```python
from build123d import *

# Parameters (mm, degrees)
F0_W          = 1422.4
F0_H          = 711.2
F0_W_2        = 654.05
F0_H_2        = 635
F1_DEPTH      = 88.9
F2_W          = 88.9
F2_H          = 88.9
F3_DEPTH      = 762
F5_W          = 1422.4
F5_H          = 711.2
F5_W_2        = 654.05
F5_H_2        = 635
F6_DEPTH      = 88.9
F7_W          = 1422.4
F7_H          = 711.2
F8_DEPTH      = 18.796
F8_DEPTH_BACK = 0.254
F9_W          = 19.05
F9_H          = 533.4
F9_W_2        = 577.85
F9_H_2        = 19.05
F10_DEPTH     = 590.804
F12_W         = 152.4
F12_H         = 635
F13_DEPTH     = 88.9
F14_W         = 654.05
F14_H         = 635
F15_DEPTH     = 19.05


with BuildPart() as f1:
    # F0 (on Top) → F1 (new body)
    with BuildSketch(Plane.XY):
        with Locations((0, -355.6)):
            Rectangle(F0_W, F0_H)
        with Locations((-346.075, -355.6)):
            Rectangle(F0_W_2, F0_H_2, mode=Mode.SUBTRACT)
        with Locations((346.075, -355.6)):
            Rectangle(F0_W_2, F0_H_2, mode=Mode.SUBTRACT)
    extrude(amount=-F1_DEPTH)

    # F2 (on Top) → F3 (join)
    with BuildSketch(Plane.XY):
        with Locations((-666.75, -44.45)):
            Rectangle(F2_W, F2_H)
        with Locations((-666.75, -666.75)):
            Rectangle(F2_W, F2_H)
        with Locations((0, -44.45)):
            Rectangle(F2_W, F2_H)
        with Locations((0, -666.75)):
            Rectangle(F2_W, F2_H)
        with Locations((666.75, -44.45)):
            Rectangle(F2_W, F2_H)
        with Locations((666.75, -666.75)):
            Rectangle(F2_W, F2_H)
    extrude(amount=-F3_DEPTH)

    # F5 (on offset) → F6 (join)
    with BuildSketch(Plane.XY.offset(-609.6)):
        with Locations((0, -355.6)):
            Rectangle(F5_W, F5_H)
        with Locations((-346.075, -355.6)):
            Rectangle(F5_W_2, F5_H_2, mode=Mode.SUBTRACT)
        with Locations((346.075, -355.6)):
            Rectangle(F5_W_2, F5_H_2, mode=Mode.SUBTRACT)
    extrude(amount=-F6_DEPTH)

    # F7 (on offset) → F8 (join, two sides)
    with BuildSketch(Plane.XY.offset(-609.6)) as f8_sk:
        with Locations((0, -355.6)):
            Rectangle(F7_W, F7_H)
    extrude(amount=F8_DEPTH)
    extrude(f8_sk.sketch, amount=-F8_DEPTH_BACK)

    # F9 (on Top) → F10 (join, through all)
    with BuildSketch(Plane.XY):
        with Locations((663.575, -355.6)):
            Rectangle(F9_W, F9_H)
        with Locations((333.375, -47.625)):
            Rectangle(F9_W_2, F9_H_2)
        with Locations((-28.575, -355.6)):
            Rectangle(F9_W, F9_H)
        with Locations((-663.575, -355.6)):
            Rectangle(F9_W, F9_H)
    extrude(amount=-F10_DEPTH)

    # F12 (on offset) → F13 (join)
    with BuildSketch(Plane.XY.offset(-381)):
        Polygon((0, 0), (-711.2, 0), (-711.2, -38.1), (-542.925, -38.1), (-542.925, -673.1), (-711.2, -673.1), (-711.2, -711.2), (0, -711.2), (0, -673.1), (-123.825, -673.1), (-123.825, -38.1), (0, -38.1), align=None)
        with Locations((-428.625, -355.6)):
            Rectangle(F12_W, F12_H, mode=Mode.SUBTRACT)
        with Locations((-238.125, -355.6)):
            Rectangle(F12_W, F12_H, mode=Mode.SUBTRACT)
    extrude(amount=-F13_DEPTH)

    # F14 (on face) → F15 (join)
    with BuildSketch(Plane.XY.offset(-381)):
        with Locations((-346.075, -355.6)):
            Rectangle(F14_W, F14_H)
    extrude(amount=-F15_DEPTH)


solid = f1.part
```
Source: CAD feature listing. Evaluate the final solid. Frame: model axes, mm. A direction names the side the tool comes from. Coordinates: 2 decimals unless noted, no trailing zeros. Order: outer loops, then holes, each group sorted by start corner. A loop starts at its lowest first (then second) coordinate and runs counter-clockwise, first axis right, second up. Notation, with made-up numbers: M -8.75,-15 L 44.25,-15 A12 cw 44.25,7 Z; hole C -32.75,-24 d5. An arc over 180 degrees is marked long. Write each question's results on one line, items separated by ' | '. Start each with the question number.
1) Section query D-D (z = -659). Return the cut outline in (x, y).
2) Section query A-A (x = -568.5). Return the cut outline in (y, z), plus the area to 3 significant figures.
3) Line query: line 1 (X direction, y = -478.5, z = -590.5); line 2 (X direction, y = -154, z = -680.5); line 3 (Z direction, x = -591, y = -585.5). Output: solid intervals per line, ascending. Write a range as from..to.
4) Access query for faces 1 (the face through (692, -352, -88.9)), 2 (the face through (-19.05, -359, -336)), 3 (the face through (622.3, -55, -702)), 4 (the face through (329, -38.1, -336)). Directions: +Z, -Z, +X, -X, +Y, -Y. A direction counts if a zero-diameter tool reaches every point of the face in a straight line with its end or side. Return the directions, or none.
5) Section query C-C (z = -69). Return the cut outline in (x, y).
6) Section query B-B (x = 213). Return the cut outline in (y, z).
7) Contact query for flat-ended pins moving along their axis: pin 1 Ø5 at (y, z) = (-369.5, -137.5) entering from -X; pin 2 Ø3 at (x, y) = (-416.5, -218.5) entering from +Z; pin 3 Ø11.5 at (x, y) = (-368.5, -688.5) entering from -Z. Output: stop coordinate, or through.
8) Draft query along Y for faces 5 (the face through (-638, -88.9, -188)), 6 (the face through (-667, -44, -762)), 7 (the face through (-168, 0, -460)), 8 (the face through (622.3, -657, -702)). Return one class per face: released by +Y, released by -Y, zero draft, split by the parting line, or undercut.
Answers:
1) outline: M -711.2,-711.2 L 711.2,-711.2 L 711.2,0 L -711.2,0 Z; hole M -673.1,-622.3 L -622.3,-622.3 L -622.3,-673.1 L -44.45,-673.1 L -44.45,-622.3 L -19.05,-622.3 L -19.05,-88.9 L -44.45,-88.9 L -44.45,-38.1 L -622.3,-38.1 L -622.3,-88.9 L -673.1,-88.9 Z; hole M 19.05,-622.3 L 44.45,-622.3 L 44.45,-673.1 L 622.3,-673.1 L 622.3,-622.3 L 673.1,-622.3 L 673.1,-88.9 L 622.3,-88.9 L 622.3,-38.1 L 44.45,-38.1 L 44.45,-88.9 L 19.05,-88.9 Z
2) outline: M -711.2,-698.5 L -673.1,-698.5 L -673.1,-609.85 L -38.1,-609.85 L -38.1,-698.5 L 0,-698.5 L 0,-590.8 L -711.2,-590.8 Z; M -711.2,-469.9 L -673.1,-469.9 L -673.1,-400.05 L -38.1,-400.05 L -38.1,-469.9 L 0,-469.9 L 0,-381 L -711.2,-381 Z; M -711.2,-88.9 L -673.1,-88.9 L -673.1,0 L -711.2,0 Z; M -38.1,-88.9 L 0,-88.9 L 0,0 L -38.1,0 Z | area: 45,900 mm^2
3) line 1: x = -673.1..-654.05, -38.1..-19.05, 654.05..673.1 | line 2: x = -711.2..-673.1, -19.05..19.05, 673.1..711.2 | line 3: z = -609.85..-590.8, -400.05..-381
4) face 1: +X | face 2: none | face 3: -Z | face 4: +Y
5) outline: M -711.2,-711.2 L 711.2,-711.2 L 711.2,0 L -711.2,0 Z; hole M -654.05,-622.3 L -622.3,-622.3 L -622.3,-673.1 L -44.45,-673.1 L -44.45,-622.3 L -38.1,-622.3 L -38.1,-88.9 L -44.45,-88.9 L -44.45,-38.1 L -622.3,-38.1 L -622.3,-88.9 L -654.05,-88.9 Z; hole M 19.05,-622.3 L 44.45,-622.3 L 44.45,-673.1 L 622.3,-673.1 L 622.3,-622.3 L 654.05,-622.3 L 654.05,-88.9 L 622.3,-88.9 L 622.3,-57.15 L 44.45,-57.15 L 44.45,-88.9 L 19.05,-88.9 Z
6) outline: M -711.2,-698.5 L -673.1,-698.5 L -673.1,-609.85 L -38.1,-609.85 L -38.1,-698.5 L 0,-698.5 L 0,-590.8 L -38.1,-590.8 L -38.1,-88.9 L 0,-88.9 L 0,0 L -57.15,0 L -57.15,-590.8 L -711.2,-590.8 Z; M -711.2,-88.9 L -673.1,-88.9 L -673.1,0 L -711.2,0 Z
7) pin 1: stops at x = -673.1 | pin 2: stops at z = -381 | pin 3: stops at z = -698.5
8) face 5: undercut | face 6: zero draft | face 7: released by +Y | face 8: undercut
